Can you work these out from the model? Positions are in its coordinate system, mm. Face numbers are marked on the shaded views. A direction names the side the tool comes from. Give positions to 0.01 mm unless a question says otherwise; leave off trailing zeros. Loops run counter-clockwise (first coordinate to the right, second up) from the corner with the lowest first, then second, coordinate; pieces in that order, holes last. Notation, with made-up numbers: M 16.5,-4.75 L 58.5,-4.75 A29 ccw 58.5,17.25 Z; hole C 15,0.25 d10. An arc over 180 degrees is marked long. Put each result on its own line as item: value. Start each with the question number.
1) For P1, Ø5, axis at y = -56, z = -44.5, coming from the +X side; P2, Ø1.9, axis at x = 40, z = -10, coming from the +Y side; P3, Ø6, axis at x = -25.5, y = -5, coming from the +Z side; P4, Ø5.5, axis at x = -18.75, z = -40, coming from the +Y side, each with a flat end and sliding along its axis, tell me the tip position at first contact or that it passes through.
2) Imagine slicing it at D-D (z = 13). Write out the boundary of the cut face in (x, y), then the cut area to 3 significant figures.
3) Please list where these lines run through material, in increasing order: line 1 along Z through (x, y) = (40, -66); line 2 along Z through (x, y) = (1, -56.5); line 3 along Y through (x, z) = (-22, 5). Write a range as from..to.
4) Imagine slicing it at B-B (y = -52). Write out the boundary of the cut face in (x, z), then the cut area to 3 significant figures.
5) Imagine slicing it at C-C (z = -10). Write out the boundary of the cut face in (x, y).
6) Imagine slicing it at A-A (x = 0). Write out the boundary of the cut face in (y, z), then the cut area to 3 significant figures.
7) If we mould it in two halves opening along X, with no side actions, what happens to the marked faces 1, 2 and 3? For each: +X half, -X half, draft (parallel to the pull), parting line (faces both ways), or undercut.
8) For the marked faces 4, 5 and 6, which set-ups out of +Z, -Z, +X, -X, +Y, -Y let a thin tool reach every point of the face, with its end or its side?
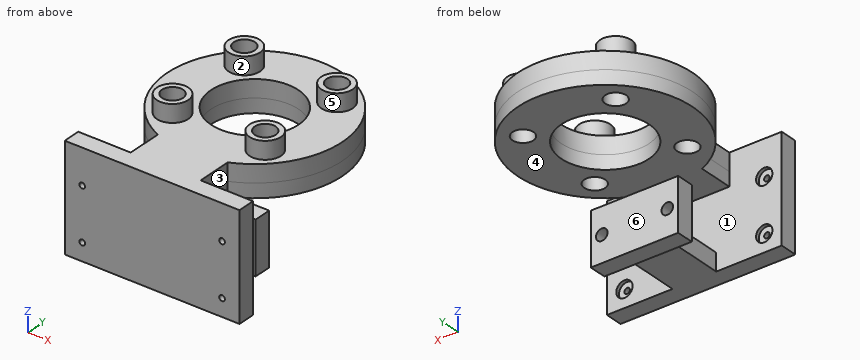
from build123d import *

# Parameters (mm, degrees)
SKETCH1_R                                    = 24.999999999999996
BOSS_EXTRUDE1_DEPTH                          = 10
BOSS_EXTRUDE2_DEPTH                          = 10
BOSS_EXTRUDE3_DEPTH                          = 10
BOSS_EXTRUDE4_DEPTH                          = 10
CUT_EXTRUDE1_REACH                           = 108.182
SKETCH5_R                                    = 6.000000000000003
SKETCH5_R_2                                  = 5.999999999999995
SKETCH5_R_3                                  = 5.999999999999999
SKETCH6_R                                    = 8.999999999999996
SKETCH6_R_2                                  = 5.999999999999995
SKETCH6_R_3                                  = 5.999999999999988
SKETCH6_R_4                                  = 9
SKETCH6_R_5                                  = 5.999999999999991
BOSS_EXTRUDE5_DEPTH                          = 10
CBORE_FOR_M3_HEX_HEAD_CAP_SCREW1_D           = 3.2
CBORE_FOR_M3_HEX_HEAD_CAP_SCREW1_CBORE_D     = 9.351
CBORE_FOR_M3_HEX_HEAD_CAP_SCREW1_CBORE_DEPTH = 2
CUT_EXTRUDE2_REACH                           = 105.242
SKETCH12_R                                   = 3.3000000000000003
CIRPATTERN1_COUNT                            = 4
BOSS_EXTRUDE6_START                          = 8
SKETCH13_R                                   = 6.000000000000003
SKETCH13_R_2                                 = 5.999999999999995
SKETCH13_R_3                                 = 5.999999999999999
SKETCH13_R_4                                 = 25
BOSS_EXTRUDE6_DEPTH                          = 8


with BuildPart() as part:
    # Sketch1 → Boss-Extrude1 (new body)
    # profile 1 of 3: a face of its own
    with BuildSketch(Plane.XY):
        with BuildLine():
            ThreePointArc((50, 0), (-27.386127875258286, 41.83300132670379), (-20.00000000000004, -45.82575694955838))
            Line((-20.000000000000004, -45.82575694955839), (20.000000000000004, -45.82575694955839))
            ThreePointArc((19.999999999999986, -45.825756949558404), (41.83300132670376, -27.38612787525834), (50, -1.225e-14))
        make_face()
        Circle(SKETCH1_R, mode=Mode.SUBTRACT)
    # profile 2 of 3: a face of its own
    with BuildSketch(Plane.XY):
        with BuildLine():
            ThreePointArc((19.999999999999986, -45.825756949558404), (-9.18e-15, -50), (-20.00000000000004, -45.82575694955838))
            Line((-20.000000000000004, -45.82575694955839), (-20, -65.82575694955838))
            Line((-20, -65.82575694955838), (20, -65.82575694955838))
            Line((20, -65.82575694955838), (20.000000000000004, -45.82575694955839))
        make_face()
    # profile 3 of 3: a face of its own
    with BuildSketch(Plane.XY):
        with BuildLine():
            Line((20.000000000000004, -45.82575694955839), (-20.000000000000004, -45.82575694955839))
            ThreePointArc((-20.00000000000004, -45.82575694955838), (-9.18e-15, -50), (19.999999999999986, -45.825756949558404))
        make_face()
    extrude(amount=BOSS_EXTRUDE1_DEPTH)

    # Sketch2 → Boss-Extrude2 (add)
    with BuildSketch(Plane.XZ.offset(65.82575694955838)):
        Polygon((-50, 10), (50, 10), (50.00000000000002, -49.99999999999999), (-49.999999999999986, -49.99999999999999), align=None)
    extrude(amount=BOSS_EXTRUDE2_DEPTH)

    # Sketch3 → Boss-Extrude3 (add)
    with BuildSketch(Plane(origin=(0, 0, -49.99999999999999), x_dir=(-1, 0, 0), z_dir=(0, 0, -1))):
        Polygon((-12.499999999999993, -75.82575694955838), (12.500000000000007, -75.82575694955838), (12.5, -21.65063509461097), (-12.5, -21.65063509461097), align=None)
    extrude(amount=-BOSS_EXTRUDE3_DEPTH)

    # Sketch4 → Boss-Extrude4 (add)
    with BuildSketch(Plane(origin=(0, -21.65063509461097, 0), x_dir=(1, 0, 0), z_dir=(0, 1, 0))):
        Polygon((-25, 24.999999999999996), (-24.999999999999996, 54.99999999999999), (25.000000000000007, 55), (25, 24.999999999999996), align=None)
    extrude(amount=-BOSS_EXTRUDE4_DEPTH)

    # Sketch5 → Cut-Extrude1 (cut, up to next)
    with BuildSketch(Plane(origin=(0, 0, 0), x_dir=(-1, 0, 0), z_dir=(0, 0, -1)), mode=Mode.PRIVATE) as cut_extrude1_sk1:
        with Locations((-26.516504294495405, 26.51650429449565)):
            Circle(SKETCH5_R)
    cut_extrude1_tool1 = extrude(cut_extrude1_sk1.sketch, amount=-CUT_EXTRUDE1_REACH, mode=Mode.PRIVATE) & part.part
    # Sketch5 → Cut-Extrude1 (cut, up to next)
    with BuildSketch(Plane(origin=(0, 0, 0), x_dir=(-1, 0, 0), z_dir=(0, 0, -1)), mode=Mode.PRIVATE) as cut_extrude1_sk2:
        with Locations((26.516504294495764, 26.5165042944953)):
            Circle(SKETCH5_R_2)
    cut_extrude1_tool2 = extrude(cut_extrude1_sk2.sketch, amount=-CUT_EXTRUDE1_REACH, mode=Mode.PRIVATE) & part.part
    # Sketch5 → Cut-Extrude1 (cut, up to next)
    with BuildSketch(Plane(origin=(0, 0, 0), x_dir=(-1, 0, 0), z_dir=(0, 0, -1)), mode=Mode.PRIVATE) as cut_extrude1_sk3:
        with Locations((26.516504294495217, -26.516504294495856)):
            Circle(SKETCH5_R)
    cut_extrude1_tool3 = extrude(cut_extrude1_sk3.sketch, amount=-CUT_EXTRUDE1_REACH, mode=Mode.PRIVATE) & part.part
    # Sketch5 → Cut-Extrude1 (cut, up to next)
    with BuildSketch(Plane(origin=(0, 0, 0), x_dir=(-1, 0, 0), z_dir=(0, 0, -1)), mode=Mode.PRIVATE) as cut_extrude1_sk4:
        with Locations((-26.516504294495945, -26.516504294495114)):
            Circle(SKETCH5_R_3)
    cut_extrude1_tool4 = extrude(cut_extrude1_sk4.sketch, amount=-CUT_EXTRUDE1_REACH, mode=Mode.PRIVATE) & part.part
    add(cut_extrude1_tool1.solids().sort_by_distance((26.516504, 26.516504, 0))[0], mode=Mode.SUBTRACT)
    add(cut_extrude1_tool2.solids().sort_by_distance((-26.516504, 26.516504, 0))[0], mode=Mode.SUBTRACT)
    add(cut_extrude1_tool3.solids().sort_by_distance((-26.516504, -26.516504, 0))[0], mode=Mode.SUBTRACT)
    add(cut_extrude1_tool4.solids().sort_by_distance((26.516504, -26.516504, 0))[0], mode=Mode.SUBTRACT)

    # Sketch6 → Boss-Extrude5 (add)
    # profile 1 of 4: a face of its own
    with BuildSketch(Plane.XY.offset(10)):
        with Locations((-26.516504294495764, 26.5165042944953)):
            Circle(SKETCH6_R)
        with Locations(Location((-26.516504294495764, 26.5165042944953, 0), (0, 0, 180))):
            Circle(SKETCH6_R_2, mode=Mode.SUBTRACT)
    # profile 2 of 4: a face of its own
    with BuildSketch(Plane.XY.offset(10)):
        with Locations((26.516504294495398, 26.51650429449567)):
            Circle(SKETCH6_R)
        with Locations(Location((26.516504294495398, 26.51650429449567, 0), (0, 0, 180))):
            Circle(SKETCH6_R_3, mode=Mode.SUBTRACT)
    # profile 3 of 4: a face of its own
    with BuildSketch(Plane.XY.offset(10)):
        with Locations((26.516504294495572, -26.51650429449549)):
            Circle(SKETCH6_R_4)
        with Locations(Location((26.516504294495572, -26.51650429449549, 0), (0, 0, 180))):
            Circle(SKETCH6_R_5, mode=Mode.SUBTRACT)
    # profile 4 of 4: a face of its own
    with BuildSketch(Plane.XY.offset(10)):
        with Locations((-26.516504294495576, -26.516504294495487)):
            Circle(SKETCH6_R)
        with Locations(Location((-26.516504294495576, -26.516504294495487, 0), (0, 0, 180))):
            Circle(SKETCH6_R_2, mode=Mode.SUBTRACT)
    boss_extrude5 = extrude(amount=BOSS_EXTRUDE5_DEPTH)

    # CBORE for M3 Hex Head Cap Screw1 (through all)
    with Locations(Plane(origin=(0, -65.82575694955838, 0), x_dir=(1, 0, 0), z_dir=(0, 1, 0))):
        with Locations((-40, 40), (40, 40), (40, 10), (-40, 10)):
            CounterBoreHole(CBORE_FOR_M3_HEX_HEAD_CAP_SCREW1_D / 2, CBORE_FOR_M3_HEX_HEAD_CAP_SCREW1_CBORE_D / 2, CBORE_FOR_M3_HEX_HEAD_CAP_SCREW1_CBORE_DEPTH)

    # Sketch12 → Cut-Extrude2 (cut, up to next)
    with BuildSketch(Plane(origin=(0, -21.65063509461097, 0), x_dir=(1, 0, 0), z_dir=(0, 1, 0)), mode=Mode.PRIVATE) as cut_extrude2_sk1:
        with Locations(Location((-18.75, 39.99999999999999, 0), (0, 0, 270))):
            Circle(SKETCH12_R)
    cut_extrude2_tool1 = extrude(cut_extrude2_sk1.sketch, amount=-CUT_EXTRUDE2_REACH, mode=Mode.PRIVATE) & part.part
    # Sketch12 → Cut-Extrude2 (cut, up to next)
    with BuildSketch(Plane(origin=(0, -21.65063509461097, 0), x_dir=(1, 0, 0), z_dir=(0, 1, 0)), mode=Mode.PRIVATE) as cut_extrude2_sk2:
        with Locations(Location((18.750000000000004, 39.99999999999999, 0), (0, 0, 270))):
            Circle(SKETCH12_R)
    cut_extrude2_tool2 = extrude(cut_extrude2_sk2.sketch, amount=-CUT_EXTRUDE2_REACH, mode=Mode.PRIVATE) & part.part
    add(cut_extrude2_tool1.solids().sort_by_distance((-18.75, -21.650635, -40))[0], mode=Mode.SUBTRACT)
    add(cut_extrude2_tool2.solids().sort_by_distance((18.75, -21.650635, -40))[0], mode=Mode.SUBTRACT)

    # CirPattern1: Boss-Extrude5 ×4 about axis
    cirpattern1_axis = Axis((0, 0, 10), (0, 0, -1))
    for i in range(1, CIRPATTERN1_COUNT):
        add(boss_extrude5.rotate(cirpattern1_axis, i * 360 / CIRPATTERN1_COUNT))

    # Sketch13 → Boss-Extrude6 (add)
    with BuildSketch(Plane(origin=(0, 0, 0), x_dir=(-1, 0, 0), z_dir=(0, 0, -1)).offset(BOSS_EXTRUDE6_START)):
        with BuildLine():
            Line((-20.00000000000004, -45.825756949558375), (-20, -65.82575694955838))
            Line((-20, -65.82575694955838), (20, -65.82575694955838))
            Line((20, -65.82575694955838), (19.999999999999982, -45.8257569495584))
            ThreePointArc((19.999999999999982, -45.8257569495584), (3.637e-14, 49.99999999999999), (-20.00000000000004, -45.825756949558375))
        make_face()
        with Locations((26.516504294495217, -26.516504294495856)):
            Circle(SKETCH13_R, mode=Mode.SUBTRACT)
        with Locations((26.516504294495764, 26.5165042944953)):
            Circle(SKETCH13_R_2, mode=Mode.SUBTRACT)
        with Locations((-26.516504294495945, -26.516504294495114)):
            Circle(SKETCH13_R_3, mode=Mode.SUBTRACT)
        with Locations((-26.516504294495405, 26.51650429449565)):
            Circle(SKETCH13_R, mode=Mode.SUBTRACT)
        Circle(SKETCH13_R_4, mode=Mode.SUBTRACT)
    extrude(amount=-BOSS_EXTRUDE6_DEPTH)


solid = part.part
Recorded:
1. P1: x = 12.5
1. P2: through
1. P3: z = 10
1. P4: y = -65.83
2. outline: C -26.52,-26.52 d18; C -26.52,26.52 d18; C 26.52,-26.52 d18; C 26.52,26.52 d18; hole C -26.52,-26.52 d12; hole C -26.52,26.52 d12; hole C 26.52,-26.52 d12; hole C 26.52,26.52 d12
2. area: 565 mm²
3. line 1: -50..-44.68, -35.32..-14.68, -5.32..10
3. line 2: -50..-40, -8..10
3. line 3: -75.83..-65.83, -44.9..-30.47, -22.57..-11.87, 11.87..22.57, 30.47..44.9
4. outline: M -20,-8 L 20,-8 L 20,10 L -20,10 Z; M -12.5,-50 L 12.5,-50 L 12.5,-40 L -12.5,-40 Z
4. area: 970 mm²
5. outline: M -50,-75.83 L -41.6,-75.83 L -41.6,-67.83 L -44.68,-67.83 L -44.68,-65.83 L -50,-65.83 Z; M -38.4,-75.83 L 38.4,-75.83 L 38.4,-67.83 L 35.32,-67.83 L 35.32,-65.83 L -35.32,-65.83 L -35.32,-67.83 L -38.4,-67.83 Z; M 41.6,-75.83 L 50,-75.83 L 50,-65.83 L 44.68,-65.83 L 44.68,-67.83 L 41.6,-67.83 Z
6. outline: M -75.83,-50 L -31.65,-50 L -31.65,-55 L -21.65,-55 L -21.65,-25 L -31.65,-25 L -31.65,-40 L -65.83,-40 L -65.83,-8 L -25,-8 L -25,10 L -75.83,10 Z; M 25,-8 L 50,-8 L 50,10 L 25,10 Z
6. area: 2,430 mm²
7. face 1: draft
7. face 2: undercut
7. face 3: +X half
8. face 4: +X, -X, +Y
8. face 5: +Z
8. face 6: -Z, +X, -X, +Y
